from build123d import *

# Parameters (mm, degrees)
F0_R     = 195
F1_DEPTH = 15


with BuildPart() as f1:
    # F0 (on Top) → F1 (new body)
    with BuildSketch(Plane.XY):
        Circle(F0_R)
        with BuildLine():
            ThreePointArc((7, 119.795659), (87.292611, 82.340755), (120, 0))
            ThreePointArc((120, 0), (87.292611, -82.340755), (7, -119.795659))
            Line((7, -119.795659), (7, -125))
            Line((7, -125), (-7, -125))
            Line((-7, -125), (-7, -119.795659))
            ThreePointArc((-7, -119.795659), (-120, 0), (-7, 119.795659))
            Line((-7, 119.795659), (-7, 125))
            Line((-7, 125), (7, 125))
            Line((7, 125), (7, 119.795659))
        make_face(mode=Mode.SUBTRACT)
    extrude(amount=F1_DEPTH)


solid = f1.part
Part model, mm, in its own coordinate system. A direction names the side the tool comes from. Give positions to 0.01 mm unless a question says otherwise; leave off trailing zeros. Loops run counter-clockwise (first coordinate to the right, second up) from the corner with the lowest first, then second, coordinate; pieces in that order, holes last. Notation, with made-up numbers: M 39.25,-29.75 L 85.25,-29.75 A29 cw 85.25,-6.75 Z; hole C 51,23.25 d1. An arc over 180 degrees is marked long. Put each result on its own line as item: value. Start each with the question number.
1) 3-axis set-ups, long thin cutter, end or side, ignore diameter. For faces 1 (the cylindrical face through (-119.973, -2.541, 7.395)), 2 (the flat face through (84, 89, 0)): which of +Z, -Z, +X, -X, +Y, -Y reach the whole face in a straight line?
2) Saw through at B-B (z = 11.5). List the corners of the cut face in (x, y), then the cut area to 3 significant figures.
3) Pull direction Y, two halves, no side cores. Call faces 3 (the flat face through (0, 125, 7)), 4 (the flat face through (84, 89, 15)), 5 (the cylindrical face through (-154.75, -118.65, 7.4)): +Y half, -Y half, draft (parallel to the pull), parting line (faces both ways), or undercut.
4) Saw through at D-D (x = -151). List the corners of the cut face in (y, z).
5) Flat gauge pins, fed straight in: pin 1 (5.5 mm diameter, centred on y = 122, z = 7.5, fed in from +X); pin 2 (2 mm diameter, centred on x = 25.5, z = 2, fed in from +Y); pin 3 (3 mm diameter, centred on x = -44.5, z = 8.5, fed in from -Y). Where does each tip first touch, or does it go through?
6) Saw through at C-C (y = 34). List the corners of the cut face in (x, z), then the cut area to 3 significant figures.
7) Saw through at A-A (x = 0). List the corners of the cut face in (y, z).
8) Probe probe 1 along Y at (x, z) = (52.5, 11.5); probe 2 along Y at (x, z) = (-21, 8); probe 3 along X at (y, z) = (121, 3.75). List the from-to ranges inside material, lowest first.
Numbers:
1. face 1: +Z, -Z
1. face 2: -Z, +X, -X, +Y, -Y
2. outline: C 0,0 d390; hole M -7,-125 L 7,-125 L 7,-119.8 A120 ccw 120,0 A120 ccw 7,119.8 L 7,125 L -7,125 L -7,119.8 A120 ccw -7,-119.8 Z
2. area: 74,100 mm^2
3. face 3: undercut
3. face 4: draft
3. face 5: parting line
4. outline: M -123.39,0 L 123.39,0 L 123.39,15 L -123.39,15 Z
5. pin 1: x = 154.29
5. pin 2: y = 193.45
5. pin 3: y = -190.2
6. outline: M -192.01,0 L -115.08,0 L -115.08,15 L -192.01,15 Z; M 115.08,0 L 192.01,0 L 192.01,15 L 115.08,15 Z
6. area: 2,310 mm^2
7. outline: M -195,0 L -125,0 L -125,15 L -195,15 Z; M 125,0 L 195,0 L 195,15 L 125,15 Z
8. probe 1: -187.8 to -107.91, 107.91 to 187.8
8. probe 2: -193.87 to -118.15, 118.15 to 193.87
8. probe 3: -152.92 to -7, 7 to 152.92
